Read the model definition and answer for the solid it produces. Units are mm, in the model's axes. A direction names the side the tool comes from. Give positions to 0.01 mm unless a question says otherwise; leave off trailing zeros. Loops run counter-clockwise (first coordinate to the right, second up) from the corner with the lowest first, then second, coordinate; pieces in that order, holes last. Notation, with made-up numbers: (54.5, -15.5) - (83.5, -15.5) arc R26 cw to (83.5, 2.5) - close; hole circle Ø4 at (61.5, 54). An arc over 180 degrees is marked (long way). Write item = value, one per line. Start each with the question number.
from build123d import *

# Parameters (mm, degrees)
SKETCH1_W           = 30
SKETCH1_H           = 26
SKETCH1_R           = 11
BOSS_EXTRUDE1_DEPTH = 3.5
SKETCH1_3_W         = 10
SKETCH1_3_H         = 20
BOSS_EXTRUDE2_DEPTH = 5
SKETCH2_R           = 2.05
CUT_EXTRUDE1_DEPTH  = 30
FILLET1_R           = 4
CHAMFER1_SIZE       = 6
SKETCH3_R           = 6.5
BOSS_EXTRUDE3_DEPTH = 1.5


with BuildPart() as part:
    # Sketch1 → Boss-Extrude1 (new, symmetric)
    with BuildSketch(Plane(origin=(0, 0, 0), x_dir=(1, 0, 0), z_dir=(0, 1, 0))):
        Rectangle(SKETCH1_W, SKETCH1_H)
        with Locations(Location((0, 0, 0), (0, 0, 270))):
            Circle(SKETCH1_R, mode=Mode.SUBTRACT)
    extrude(amount=BOSS_EXTRUDE1_DEPTH, both=True)

    # Sketch1<3> → Boss-Extrude2 (add, symmetric)
    with BuildSketch(Plane(origin=(0, 0, 0), x_dir=(1, 0, 0), z_dir=(0, 1, 0))):
        with Locations((-20, 0)):
            Rectangle(SKETCH1_3_W, SKETCH1_3_H)
        with Locations((20, 0)):
            Rectangle(SKETCH1_3_W, SKETCH1_3_H)
    extrude(amount=BOSS_EXTRUDE2_DEPTH, both=True)

    # Sketch2 → Cut-Extrude1 (cut)
    with BuildSketch(Plane(origin=(0, 0, -10), x_dir=(-1, 0, 0), z_dir=(0, 0, -1))):
        with Locations((-20, 0)):
            Circle(SKETCH2_R)
        with Locations((20, 0)):
            Circle(SKETCH2_R)
    extrude(amount=-CUT_EXTRUDE1_DEPTH, mode=Mode.SUBTRACT)

    # Fillet1
    fillet1_edges = [part.edges().sort_by_distance(p)[0] for p in [
        (-25, -5, 0),
        (-25, 5, 0),
        (25, 5, 0),
        (25, -5, 0),
    ]]
    fillet(fillet1_edges, radius=FILLET1_R)

    # Chamfer1
    # the kernel refuses this chamfer: 6 mm, written as the material it takes off along each edge
    with BuildSketch(Plane(origin=(15, -18.930097928, -13), x_dir=(0.02749587661058649, 0, 0.9996219169112968), z_dir=(0, 1, 0))) as chamfer1_piece_1_section:
        Polygon((CHAMFER1_SIZE * 0.999621916911, -CHAMFER1_SIZE * 0.0274958766106), (-CHAMFER1_SIZE * 0.0274958766106, -CHAMFER1_SIZE * 0.999621916911), (0, 0), align=None)
    chamfer1_piece_1 = extrude(amount=37.860195856, mode=Mode.PRIVATE)
    chamfer1_piece_1 = split(chamfer1_piece_1, bisect_by=Plane(origin=(12.639593495, 0, -10), z_dir=(0, 0, -1)), keep=Keep.TOP, mode=Mode.PRIVATE)
    add(chamfer1_piece_1, mode=Mode.SUBTRACT)
    with BuildSketch(Plane(origin=(15, 18.930097928, 13), x_dir=(0.02749587661058649, 0, -0.9996219169112968), z_dir=(0, -1, 0))) as chamfer1_piece_2_section:
        Polygon((CHAMFER1_SIZE * 0.999621916911, -CHAMFER1_SIZE * 0.0274958766106), (-CHAMFER1_SIZE * 0.0274958766106, -CHAMFER1_SIZE * 0.999621916911), (0, 0), align=None)
    chamfer1_piece_2 = extrude(amount=37.860195856, mode=Mode.PRIVATE)
    chamfer1_piece_2 = split(chamfer1_piece_2, bisect_by=Plane(origin=(12.639593495, 0, 10), z_dir=(0, 0, 1)), keep=Keep.TOP, mode=Mode.PRIVATE)
    add(chamfer1_piece_2, mode=Mode.SUBTRACT)
    with BuildSketch(Plane(origin=(-15, 18.930097928, 13), x_dir=(0.9996219169112969, 0, 0.02749587661058649), z_dir=(0, -1, 0))) as chamfer1_piece_3_section:
        Polygon((CHAMFER1_SIZE * 0.999621916911, -CHAMFER1_SIZE * 0.0274958766106), (-CHAMFER1_SIZE * 0.0274958766106, -CHAMFER1_SIZE * 0.999621916911), (0, 0), align=None)
    chamfer1_piece_3 = extrude(amount=37.860195856, mode=Mode.PRIVATE)
    chamfer1_piece_3 = split(chamfer1_piece_3, bisect_by=Plane(origin=(-12.639593495, 0, 10), z_dir=(0, 0, 1)), keep=Keep.TOP, mode=Mode.PRIVATE)
    add(chamfer1_piece_3, mode=Mode.SUBTRACT)
    with BuildSketch(Plane(origin=(-15, -18.930097928, -13), x_dir=(0.9996219169112969, 0, -0.02749587661058649), z_dir=(0, 1, 0))) as chamfer1_piece_4_section:
        Polygon((CHAMFER1_SIZE * 0.999621916911, -CHAMFER1_SIZE * 0.0274958766106), (-CHAMFER1_SIZE * 0.0274958766106, -CHAMFER1_SIZE * 0.999621916911), (0, 0), align=None)
    chamfer1_piece_4 = extrude(amount=37.860195856, mode=Mode.PRIVATE)
    chamfer1_piece_4 = split(chamfer1_piece_4, bisect_by=Plane(origin=(-12.639593495, 0, -10), z_dir=(0, 0, -1)), keep=Keep.TOP, mode=Mode.PRIVATE)
    add(chamfer1_piece_4, mode=Mode.SUBTRACT)

    # Sketch3 → Boss-Extrude3 (add)
    with BuildSketch(Plane(origin=(0, 3.5, 0), x_dir=(1, 0, 0), z_dir=(0, 1, 0))):
        Polygon((15, -10), (15, 10), (12, 10), (9, 13), (-9, 13), (-12, 10), (-15, 10), (-15, -10), (-12, -10), (-9, -13), (9, -13), (12, -10), align=None)
        with Locations(Location((0, 0, 0), (0, 0, 270))):
            Circle(SKETCH3_R, mode=Mode.SUBTRACT)
    extrude(amount=BOSS_EXTRUDE3_DEPTH)


solid = part.part
1. A cutting plane is placed at D-D on z = -7. Give the vertices of the cut face in (x, y), and give its area (3 significant figures).
2. A tool of negligible diameter and unlimited length cuts with its end or side. For faces 4 (the flat face through (-17, 0, 10)), 5 (the flat face through (17, 0, 10)), 6 (the flat face through (-15, -4, 0)), 7 (the flat face through (5, 3.5, 5)), from which of +Z, -Z, +X, -X, +Y, -Y can it reach the whole face along a straight path? Write none if from no direction.
3. Consider line 1 along Y through (x, z) = (-20, -4.75); line 2 along X through (y, z) = (-1.75, 5); line 3 along X through (y, z) = (1.25, 0). Determine where each line is inside the solid, lowest interval first. Write a range as [from, to].
4. A cutting plane is placed at A-A on y = 0. Give the vertices of the cut face in (x, z), and give its area (3 significant figures).
5. A cutting plane is placed at B-B on z = -1.5. Give the vertices of the cut face in (x, y), and give its area (3 significant figures).
6. For a pull along Y with two mould halves and no side action, classify faces 1 (the cylindrical face through (-17.95, 0.09, -0.14)), 2 (the cylindrical face through (-10.74, -0.05, -2.38)), 3 (the cylindrical face through (23.797, -3.859, -0.14)) as released by +Y, released by -Y, zero draft, split by the parting line, or undercut.
7. Given P1, Ø1.6, axis at y = -4.5, z = -0.5, coming from the -X side; P2, Ø11, axis at x = -3, z = 1.5, coming from the -Y side; P3, Ø1, axis at x = -13.5, y = -0.5, coming from the +Z side, each flat-ended and moving along its own axis, determine where each tip first touches the part or whether it passes through.
8. A cutting plane is placed at C-C on x = 20. Give the vertices of the cut face in (y, z), and give its area (3 significant figures).
Reply:
q1.outline = (-25, -1) arc R4 ccw to (-21, -5) - (-15, -5) - (-15, -3.5) - (-8.49, -3.5) - (-8.49, 3.5) - (8.49, 3.5) - (8.49, -3.5) - (15, -3.5) - (15, -5) - (21, -5) arc R4 ccw to (25, -1) - (25, 1) arc R4 ccw to (21, 5) - (-21, 5) arc R4 ccw to (-25, 1) - close; hole circle Ø4.1 at (-20, 0); hole circle Ø4.1 at (20, 0)
q1.area = 296 mm^2
q2.face_4 = +Z, -X, +Y, -Y
q2.face_5 = +Z, +X, +Y, -Y
q2.face_6 = +Z, -Z, -Y
q2.face_7 = -Y
q3.line_1 = [-5, -2.05], [2.05, 5]
q3.line_2 = [-24.93, -21.07], [-18.93, -9.8], [9.8, 18.93], [21.07, 24.93]
q3.line_3 = [-24.99, -21.62], [-18.38, -11], [11, 18.38], [21.62, 24.99]
q4.outline = (-25, -10) - (-22.05, -10) - (-22.05, 10) - (-25, 10) - close; (-17.95, -10) - (-12, -10) - (-9, -13) - (9, -13) - (12, -10) - (17.95, -10) - (17.95, 10) - (12, 10) - (9, 13) - (-9, 13) - (-12, 10) - (-17.95, 10) - close; (22.05, -10) - (25, -10) - (25, 10) - (22.05, 10) - close; hole circle Ø22 at (0, 0)
q4.area = 582 mm^2
q5.outline = (-25, -1) arc R4 ccw to (-21, -5) - (-15, -5) - (-15, -3.5) - (-10.9, -3.5) - (-10.9, 3.5) - (-6.32, 3.5) - (-6.32, 5) - (-21, 5) arc R4 ccw to (-25, 1) - close; (6.32, 3.5) - (10.9, 3.5) - (10.9, -3.5) - (15, -3.5) - (15, -5) - (21, -5) arc R4 ccw to (25, -1) - (25, 1) arc R4 ccw to (21, 5) - (6.32, 5) - close; hole circle Ø4.1 at (-20, 0); hole circle Ø4.1 at (20, 0)
q5.area = 243 mm^2
q6.face_1 = undercut
q6.face_2 = zero draft
q6.face_3 = released by -Y
q7.P1 = -23.95
q7.P2 = 3.5
q7.P3 = 10
q8.outline = (-5, -10) - (-2.05, -10) - (-2.05, 10) - (-5, 10) - close; (2.05, -10) - (5, -10) - (5, 10) - (2.05, 10) - close
q8.area = 118 mm^2
